```python
from build123d import *

# Parameters (mm, degrees)
BOSS_EXTRUDE1_DEPTH = 3


with BuildPart() as part:
    # Sketch1 → Boss-Extrude1 (new body)
    with BuildSketch(Plane.XY):
        with BuildLine():
            Line((278.748942769, 1025.68174137), (277.072289062, 1025.68174137))
            ThreePointArc((277.072289062, 1025.68174137), (276.81576773, 1025.613006812), (276.627980847, 1025.425220446))
            ThreePointArc((276.627980847, 1025.425220446), (275.820896535, 1025.31896689), (275.927149562, 1026.126051271))
            ThreePointArc((275.927149562, 1026.126051271), (276.114935991, 1026.313838161), (276.183670574, 1026.570359537))
            Line((276.183670574, 1026.570359537), (276.183670574, 1031.88000541))
            Line((276.183670574, 1031.88000541), (273.383670574, 1031.88000541))
            Line((273.383670574, 1031.88000541), (273.383670574, 1030.53000541))
            Line((273.383670574, 1030.53000541), (269.183670574, 1030.53000541))
            Line((269.183670574, 1030.53000541), (269.183670574, 1031.88000541))
            Line((269.183670574, 1031.88000541), (266.183670574, 1031.88000541))
            Line((266.183670574, 1031.88000541), (266.183670574, 1035.08000541))
            Line((266.183670574, 1035.08000541), (269.183670574, 1035.08000541))
            Line((269.183670574, 1035.08000541), (269.183670574, 1036.43000541))
            Line((269.183670574, 1036.43000541), (273.383670574, 1036.43000541))
            Line((273.383670574, 1036.43000541), (273.383670574, 1035.08000541))
            Line((273.383670574, 1035.08000541), (276.183670574, 1035.08000541))
            Line((276.183670574, 1035.08000541), (276.183670574, 1040.389649836))
            ThreePointArc((276.183670574, 1040.389649836), (276.114935781, 1040.646171575), (275.927148835, 1040.833958522))
            ThreePointArc((275.927148835, 1040.833958522), (275.820893173, 1041.641043417), (276.627978373, 1041.534790067))
            ThreePointArc((276.627978373, 1041.534790067), (276.815765346, 1041.347004134), (277.072286505, 1041.278269871))
            Line((277.072286505, 1041.278269871), (278.748941322, 1041.278269871))
            ThreePointArc((278.748941322, 1041.278269871), (279.111717845, 1041.428536827), (279.2619848, 1041.791313349))
            Line((279.2619848, 1041.791313349), (279.2619848, 1046.92174608))
            ThreePointArc((279.2619848, 1046.92174608), (279.111717845, 1047.284522602), (278.748941322, 1047.434789558))
            Line((278.748941322, 1047.434789558), (277.072287615, 1047.434789558))
            ThreePointArc((277.072287615, 1047.434789558), (276.815766284, 1047.366055), (276.6279794, 1047.178268634))
            ThreePointArc((276.6279794, 1047.178268634), (275.820895088, 1047.072015078), (275.927148115, 1047.879099459))
            ThreePointArc((275.927148115, 1047.879099459), (276.114934137, 1048.066885643), (276.183669127, 1048.323406094))
            Line((276.183669127, 1048.323406094), (276.183669127, 1059.132180233))
            Line((276.183669127, 1059.132180233), (265.374902832, 1059.132180233))
            ThreePointArc((265.374902832, 1059.132180233), (265.118381093, 1059.06344544), (264.930594147, 1058.875658494))
            ThreePointArc((264.930594147, 1058.875658494), (264.12351003, 1058.769403455), (264.229761575, 1059.576488032))
            ThreePointArc((264.229761575, 1059.576488032), (264.417547508, 1059.764275005), (264.486281771, 1060.020796163))
            Line((264.486281771, 1060.020796163), (264.486281771, 1061.697450981))
            ThreePointArc((264.486281771, 1061.697450981), (264.336014816, 1062.060227503), (263.973238293, 1062.210494459))
            Line((263.973238293, 1062.210494459), (258.842805647, 1062.210494459))
            ThreePointArc((258.842805647, 1062.210494459), (258.480029457, 1062.060227836), (258.329762168, 1061.697451923))
            Line((258.329762168, 1061.697451923), (258.329762168, 1060.020799457))
            ThreePointArc((258.329762168, 1060.020799457), (258.398497036, 1059.764277588), (258.586284167, 1059.576490622))
            ThreePointArc((258.586284167, 1059.576490622), (258.692539677, 1058.769406567), (257.885455039, 1058.875657641))
            ThreePointArc((257.885455039, 1058.875657641), (257.697667956, 1059.063443464), (257.441146757, 1059.132177578))
            Line((257.441146757, 1059.132177578), (252.173247105, 1059.132177578))
            Line((252.173247105, 1059.132177578), (252.173247105, 1056.332177578))
            Line((252.173247105, 1056.332177578), (253.481501818, 1056.332177578))
            Line((253.481501818, 1056.332177578), (253.481501818, 1052.132177578))
            Line((253.481501818, 1052.132177578), (252.173247105, 1052.132177578))
            Line((252.173247105, 1052.132177578), (252.173247105, 1049.132177578))
            Line((252.173247105, 1049.132177578), (248.889756531, 1049.132177578))
            Line((248.889756531, 1049.132177578), (248.889756531, 1051.949568882))
            Line((248.889756531, 1051.949568882), (247.581501818, 1051.949568882))
            Line((247.581501818, 1051.949568882), (247.581501818, 1056.332177578))
            Line((247.581501818, 1056.332177578), (248.889756531, 1056.332177578))
            Line((248.889756531, 1056.332177578), (248.889756531, 1059.132177578))
            Line((248.889756531, 1059.132177578), (243.621854827, 1059.132177578))
            ThreePointArc((243.621854827, 1059.132177578), (243.365333088, 1059.063442785), (243.177546141, 1058.875655838))
            ThreePointArc((243.177546141, 1058.875655838), (242.370461246, 1058.769400177), (242.476714596, 1059.576485377))
            ThreePointArc((242.476714596, 1059.576485377), (242.664500529, 1059.764272349), (242.733234792, 1060.020793508))
            Line((242.733234792, 1060.020793508), (242.733234792, 1061.697448325))
            ThreePointArc((242.733234792, 1061.697448325), (242.582967836, 1062.060224848), (242.220191314, 1062.210491804))
            Line((242.220191314, 1062.210491804), (237.089758668, 1062.210491804))
            ThreePointArc((237.089758668, 1062.210491804), (236.726982478, 1062.060225181), (236.576715189, 1061.697449267))
            Line((236.576715189, 1061.697449267), (236.576715189, 1060.020796683))
            ThreePointArc((236.576715189, 1060.020796683), (236.645450027, 1059.764274865), (236.833237085, 1059.576487907))
            ThreePointArc((236.833237085, 1059.576487907), (236.939492407, 1058.769403827), (236.132407793, 1058.875655089))
            ThreePointArc((236.132407793, 1058.875655089), (235.944620754, 1059.063440956), (235.688099571, 1059.132175129))
            Line((235.688099571, 1059.132175129), (226.93149811, 1059.132175129))
            Line((226.93149811, 1059.132175129), (226.93149811, 1058.427981397))
            ThreePointArc((226.93149811, 1058.427981397), (227.55634793, 1055.286649403), (229.335769658, 1052.623556781))
            Line((229.335769658, 1052.623556781), (269.675051729, 1012.284272653))
            ThreePointArc((269.675051729, 1012.284272653), (272.338145025, 1010.504850709), (275.479477777, 1009.880001213))
            Line((275.479477777, 1009.880001213), (276.183670574, 1009.880001213))
            Line((276.183670574, 1009.880001213), (276.183670574, 1018.636602674))
            ThreePointArc((276.183670574, 1018.636602674), (276.114935781, 1018.893124413), (275.927148835, 1019.08091136))
            ThreePointArc((275.927148835, 1019.08091136), (275.820893173, 1019.887996255), (276.627978373, 1019.781742905))
            ThreePointArc((276.627978373, 1019.781742905), (276.815765346, 1019.593956972), (277.072286504, 1019.525222709))
            Line((277.072286504, 1019.525222709), (278.748941322, 1019.525222709))
            ThreePointArc((278.748941322, 1019.525222709), (279.111717844, 1019.675489665), (279.2619848, 1020.038266187))
            Line((279.2619848, 1020.038266187), (279.2619848, 1025.168697892))
            ThreePointArc((279.2619848, 1025.168697892), (279.111718356, 1025.531473903), (278.748942769, 1025.68174137))
        make_face()
    extrude(amount=BOSS_EXTRUDE1_DEPTH)


solid = part.part
```
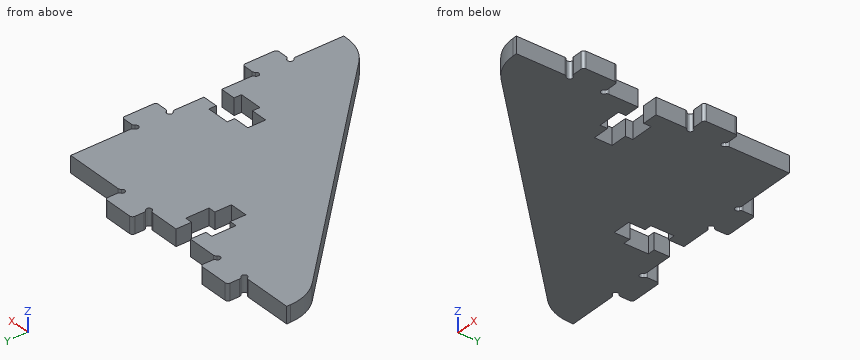
CAD build for the part. Positions are in the model's coordinates, mm. Coordinates: 2 decimals unless noted, no trailing zeros. Write each loop counter-clockwise with the first axis right and the second up, starting at its lowest first coordinate (ties: lowest second). Pieces come first, ordered by that corner, then holes.
(1) Cut at B-B, the plane y = 1043.5. List the corners of the cut face in (x, z), and give its area (3 significant figures).
(2) Drill centre lines: probe 1 along Y at (x, z) = (230, 1.55); probe 2 along X at (y, z) = (1055, 0.45); probe 3 along Y at (x, z) = (252.5, 2.55). Where is each one in solid material? Low to high.
(3) Flat gauge pins, fed straight in: pin 1 (1 mm diameter, centred on y = 1055.5, z = 1, fed in from -X); pin 2 (0.8 mm diameter, centred on y = 1061, z = 1.5, fed in from -X); pin 3 (0.7 mm diameter, centred on y = 1035.5, z = 2, fed in from -X). Where does each tip first touch, or does it go through?
(4) Cut at C-C, the plane x = 245.5. List the corners of the cut face in (y, z), and give its area (3 significant figures).
(5) Cut at A-A, the plane x = 271. List the corners of the cut face in (y, z).
Geometry says:
1. outline: (238.46, 0) - (279.26, 0) - (279.26, 3) - (238.46, 3) - close
1. area: 122 mm2
2. probe 1: y = 1051.96 to 1059.13
2. probe 2: x = 227.68 to 247.58, 253.48 to 276.18
2. probe 3: y = 1029.46 to 1052.13, 1056.33 to 1059.13
3. pin 1: stops at x = 227.3
3. pin 2: stops at x = 236.58
3. pin 3: stops at x = 246.11
4. outline: (1036.46, 0) - (1059.13, 0) - (1059.13, 3) - (1036.46, 3) - close
4. area: 68.0 mm2
5. outline: (1011.21, 0) - (1030.53, 0) - (1030.53, 3) - (1011.21, 3) - close; (1036.43, 0) - (1059.13, 0) - (1059.13, 3) - (1036.43, 3) - close
